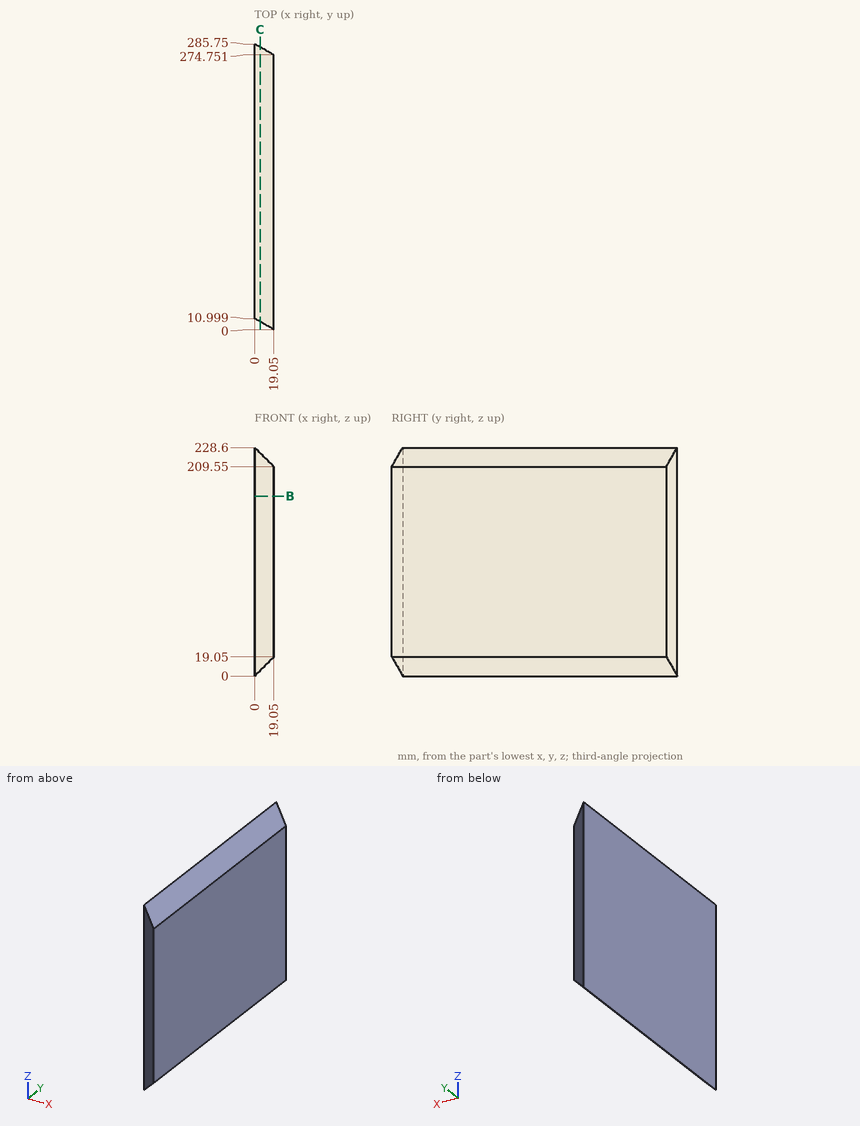
Print and shaded views of the part. All mm, measured from the part's lowest x, y and z. Coordinates: 2 decimals unless noted, no trailing zeros. Write each loop counter-clockwise with the first axis right and the second up, starting at its lowest first coordinate (ties: lowest second). Pieces come first, ordered by that corner, then holes. Notation, with made-up numbers: M 71,55 L 102,55 A9 cw 102,59 Z; hole C 70.25,71 d10. An arc over 180 degrees is marked long. Return JSON: item names as keys, results as strings.
1. Probe L1, parallel to Y at x = 17, z = 43 (1 decimal); L2, parallel to Y at x = 14.75, z = 110 (1 decimal); L3, parallel to Z at x = 4.75, y = 31. List the from-to ranges inside material, lowest first.
Determined:
{"L1": "1.2 to 275.9", "L2": "2.5 to 277.2", "L3": "4.75 to 223.85"}
2. Saw through at C-C, the plane x = 5.5. Write the cut outline in (y, z) (1 decimal).
Determined:
{"outline": "M 7.8,5.5 L 282.6,5.5 L 282.6,223.1 L 7.8,223.1 Z"}
3. Flat gauge pins, fed straight in: pin 1 Ø3 at (x, y) = (4, 112.5) entering from -Z; pin 2 Ø1.5 at (x, y) = (3.5, 182) entering from +Z; pin 3 Ø8 at (x, z) = (2, 62) entering from -Y (1 decimal). Where does each tip first touch, or does it go through?
Determined:
{"pin 1": "z = 2.5", "pin 2": "z = 225.85", "pin 3": "y = 7.5"}
4. Saw through at B-B, the plane z = 180. Write the cut outline in (x, y), then the cut area to 3 significant figures.
Determined:
{"outline": "M 0,11 L 19.05,0 L 19.05,274.75 L 0,285.75 Z", "area": "5,230 mm²"}
